Check sheet for the modelled part. Datum: model origin and axes. Units: mm. A direction names the side the tool comes from. Round coordinates to 2 decimals unless told otherwise and drop trailing zeros. Order: outer loops, then holes, each group sorted by start corner. A loop starts at its lowest first (then second) coordinate and runs counter-clockwise, first axis right, second up.
Q1. Cross-section at B-B on y = -62. Record the cut outline in (x, z).
Q2. Cross-section at D-D on y = -26. Record the cut outline in (x, z), then the cut area to 3 significant figures.
Q3. Set-up check for faces 4 (the flat face through (29, -14, 10)), 5 (the flat face through (98, 6, 2)), 6 (the cylindrical face through (-3.94, -45, -15.57)): record each of +Z, -Z, +X, -X, +Y, -Y from which the full face is reachable in a straight line by a thin tool's end or side.
Q4. Cross-section at A-A on x = 80.25. Record the cut outline in (y, z).
Q5. Scan lines: probe 1 along X at (y, z) = (8, 0); probe 2 along Z at (x, y) = (100.5, 4); probe 3 along X at (y, z) = (3, 9). Record each from-to range of solid material in increasing order.
Q6. Mould release check, pull along X, two halves, no side actions. Record for faces 1 (the flat face through (-4, -83, 0)), 2 (the cylindrical face through (-6.425, -33.544, -13.451)), 3 (the cylindrical face through (86.095, 7.521, -10.617)): +X half, -X half, draft (parallel to the pull), parting line (faces both ways), or undercut.
Q7. Depth check by flat-ended pin: P1, Ø15, axis at x = 37.5, y = -7.5, coming from the -Z side; P2, Ø3.5, axis at x = 90, z = -9.75, coming from the -Y side; P3, Ø12.5, axis at y = -70.5, z = -9.5, coming from the +X side. Enter the tip coordinate at first touch or a pass-through.
Q8. Cross-section at C-C on z = -15.5. Record the cut outline in (x, y), then the cut area to 3 significant figures.
from build123d import *

# Parameters (mm, degrees)
SKETCH_1_R           = 1.6
SKETCH_1_R_2         = 2.1
EXTRUDE_2_DEPTH      = 9
SKETCH_3_R           = 4
CUT_EXTRUDE_2_DEPTH  = 3
SKETCH_4_W           = 22.834782432
SKETCH_4_H           = 34.021608207
CUT_EXTRUDE_3_DEPTH  = 10
SKETCH_5_W           = 8
SKETCH_5_H           = 34
SKETCH_5_R           = 1.6
EXTRUDE_3_DEPTH      = 6
SKETCH_6_R           = 3.5
CUT_EXTRUDE_4_DEPTH  = 3
CUT_EXTRUDE_5_DEPTH  = 13
EXTRUDE_4_DEPTH      = 35
CUT_EXTRUDE_6_DEPTH  = 40
SKETCH_10_W          = 118.393769374
SKETCH_10_H          = 1
CUT_EXTRUDE_7_DEPTH  = 40
SKETCH_11_W          = 80.430163382
SKETCH_11_H          = 7.146133908
CUT_EXTRUDE_8_DEPTH  = 40
EXTRUDE_5_DEPTH      = 34
SKETCH_14_W          = 42
SKETCH_14_H          = 42
EXTRUDE_6_DEPTH      = 8
SKETCH_13_R          = 1.5
SKETCH_13_R_2        = 12
CUT_EXTRUDE_10_DEPTH = 8
SKETCH_15_W          = 89.303663432
SKETCH_15_H          = 7
SKETCH_15_H_2        = 10
EXTRUDE_7_DEPTH      = 4
FILLET_1_R           = 10
FILLET_2_R           = 10
FILLET_3_R           = 3


with BuildPart() as part:
    # 草图1 → 凸台-拉伸2 (new body)
    with BuildSketch(Plane(origin=(0, 0, 0), x_dir=(1, 0, 0), z_dir=(0, 1, 0))):
        with BuildLine():
            Line((0, 17), (90, 17))
            ThreePointArc((90, 17), (107, 0), (90, -17))
            Line((90, -17), (0, -17))
            ThreePointArc((0, -17), (-17, 0), (0, 17))
        make_face()
        with Locations(Location((90, 0, 0), (0, 0, 270))):
            Circle(SKETCH_1_R, mode=Mode.SUBTRACT)
        with Locations(Location((90, 9.75, 0), (0, 0, 270))):
            Circle(SKETCH_1_R, mode=Mode.SUBTRACT)
        with Locations(Location((99.75, 0, 0), (0, 0, 270))):
            Circle(SKETCH_1_R_2, mode=Mode.SUBTRACT)
        with Locations(Location((90, -9.75, 0), (0, 0, 270))):
            Circle(SKETCH_1_R, mode=Mode.SUBTRACT)
        with Locations(Location((80.25, 0, 0), (0, 0, 270))):
            Circle(SKETCH_1_R_2, mode=Mode.SUBTRACT)
    extrude(amount=EXTRUDE_2_DEPTH)

    # 草图3 → 切除-拉伸2 (cut)
    with BuildSketch(Plane(origin=(0, 9, 0), x_dir=(1, 0, 0), z_dir=(0, 1, 0))):
        with Locations(Location((90, 9.75, 0), (0, 0, 270))):
            Circle(SKETCH_3_R)
        with Locations(Location((99.75, 0, 0), (0, 0, 270))):
            Circle(SKETCH_3_R)
        with Locations(Location((90, -9.75, 0), (0, 0, 270))):
            Circle(SKETCH_3_R)
        with Locations(Location((80.25, 0, 0), (0, 0, 270))):
            Circle(SKETCH_3_R)
    extrude(amount=-CUT_EXTRUDE_2_DEPTH, mode=Mode.SUBTRACT)

    # 草图4 → 切除-拉伸3 (cut)
    with BuildSketch(Plane(origin=(0, 9, 0), x_dir=(1, 0, 0), z_dir=(0, 1, 0))):
        with Locations((-11.417391216, 0.010804103)):
            Rectangle(SKETCH_4_W, SKETCH_4_H)
    extrude(amount=-CUT_EXTRUDE_3_DEPTH, mode=Mode.SUBTRACT)

    # 草图5 → 凸台-拉伸3 (add)
    with BuildSketch(Plane(origin=(0, 9, 0), x_dir=(1, 0, 0), z_dir=(0, 1, 0))):
        with Locations((-4, 0)):
            Rectangle(SKETCH_5_W, SKETCH_5_H)
        with Locations(Location((-4, 10, 0), (0, 0, 270))):
            Circle(SKETCH_5_R, mode=Mode.SUBTRACT)
        with Locations(Location((-4, 0, 0), (0, 0, 270))):
            Circle(SKETCH_5_R, mode=Mode.SUBTRACT)
        with Locations(Location((-4, -10, 0), (0, 0, 270))):
            Circle(SKETCH_5_R, mode=Mode.SUBTRACT)
    extrude(amount=-EXTRUDE_3_DEPTH)

    # 草图6 → 切除-拉伸4 (cut)
    with BuildSketch(Plane(origin=(0, 9, 0), x_dir=(1, 0, 0), z_dir=(0, 1, 0))):
        with Locations(Location((-4, 10, 0), (0, 0, 270))):
            Circle(SKETCH_6_R)
        with Locations(Location((-4, 0, 0), (0, 0, 270))):
            Circle(SKETCH_6_R)
        with Locations(Location((-4, -10, 0), (0, 0, 270))):
            Circle(SKETCH_6_R)
    extrude(amount=-CUT_EXTRUDE_4_DEPTH, mode=Mode.SUBTRACT)

    # 草图7 → 切除-拉伸5 (cut)
    with BuildSketch(Plane(origin=(0, 9, 0), x_dir=(1, 0, 0), z_dir=(0, 1, 0))):
        with BuildLine():
            Line((68.25, -4), (7, -4))
            ThreePointArc((7, -4), (3, 0), (7, 4))
            Line((7, 4), (68.25, 4))
            ThreePointArc((68.25, 4), (72.25, 0), (68.25, -4))
        make_face()
    extrude(amount=-CUT_EXTRUDE_5_DEPTH, mode=Mode.SUBTRACT)

    # 草图8 → 凸台-拉伸4 (add)
    with BuildSketch(Plane.XY.offset(17)):
        Polygon((0, -83), (0, -41), (72.080145507, 0), (58.442959142, 0), (-8, -37.793504795), (-8, -41), (-8, -83), align=None)
    extrude(amount=-EXTRUDE_4_DEPTH)

    # 草图9 → 切除-拉伸6 (cut)
    with BuildSketch(Plane.XY.offset(17)):
        Polygon((58.442959142, 0), (68.123155874, 9), (-8, 9), (-8, 0), align=None)
    extrude(amount=-CUT_EXTRUDE_6_DEPTH, mode=Mode.SUBTRACT)

    # 草图10 → 切除-拉伸7 (cut)
    with BuildSketch(Plane(origin=(27.096230432, -29.144093474, 0), x_dir=(0.7323691027025148, 0.6809078479550029, 0), z_dir=(-0.6809078479550029, 0.7323691027025148, 0))):
        with Locations((-3.177419515, 17.5)):
            Rectangle(SKETCH_10_W, SKETCH_10_H)
    extrude(amount=-CUT_EXTRUDE_7_DEPTH, mode=Mode.SUBTRACT)

    # 草图11 → 切除-拉伸8 (cut)
    with BuildSketch(Plane(origin=(17.620285002, -30.977383092, 0), x_dir=(0.8692214499653501, 0.49442296763007937, 0), z_dir=(0.49442296763007937, -0.8692214499653501, 0))):
        with Locations((12.899580295, -20.573066954)):
            Rectangle(SKETCH_11_W, SKETCH_11_H)
    extrude(amount=-CUT_EXTRUDE_8_DEPTH, mode=Mode.SUBTRACT)

    # 草图12 → 凸台-拉伸5 (add)
    with BuildSketch(Plane.XY.offset(17)):
        Polygon((72.080145507, 0), (72.080145507, 9), (68.123155874, 9), (54.780591243, -2.083196181), (58.114256966, -7.94395497), align=None)
    extrude(amount=-EXTRUDE_5_DEPTH)

    # 草图14 → 凸台-拉伸6 (add)
    with BuildSketch(Plane.ZY.offset(8)):
        with Locations((0, -62)):
            Rectangle(SKETCH_14_W, SKETCH_14_H)
    extrude(amount=-EXTRUDE_6_DEPTH)

    # 草图13 → 切除-拉伸10 (cut)
    with BuildSketch(Plane(origin=(0, 0, 0), x_dir=(0, 0, -1), z_dir=(1, 0, 0))):
        with Locations(Location((-15.5, -46.5, 0), (0, 0, 90))):
            Circle(SKETCH_13_R)
        with Locations(Location((15.5, -46.5, 0), (0, 0, 270))):
            Circle(SKETCH_13_R)
        with Locations(Location((15.5, -77.5, 0), (0, 0, 90))):
            Circle(SKETCH_13_R)
        with Locations(Location((-15.5, -77.5, 0), (0, 0, 270))):
            Circle(SKETCH_13_R)
        with Locations(Location((0, -62, 0), (0, 0, 90))):
            Circle(SKETCH_13_R_2)
    extrude(amount=-CUT_EXTRUDE_10_DEPTH, mode=Mode.SUBTRACT)

    # 草图15 → 凸台-拉伸7 (add)
    with BuildSketch(Plane(origin=(14.286619279, -25.116624303, 0), x_dir=(0.86922144996535, 0.4944229676300795, 0), z_dir=(-0.4944229676300795, 0.86922144996535, 0))):
        with Locations((19.012083318, 13.5)):
            Rectangle(SKETCH_15_W, SKETCH_15_H)
        with Locations((19.012083318, 0)):
            Rectangle(SKETCH_15_W, SKETCH_15_H_2)
        with Locations((19.012083318, -13.5)):
            Rectangle(SKETCH_15_W, SKETCH_15_H)
    extrude(amount=EXTRUDE_7_DEPTH)

    # 圆角1
    # the kernel refuses this fillet: 10 mm, written as the material it takes off along each edge
    with BuildSketch(Plane(origin=(67.646967944, 9.837163299, -27.704780935), x_dir=(-0.8692214499653496, -0.4944229676300802, 0), z_dir=(0, 0, 1))) as fillet_1_piece_1:
        with BuildLine():
            CenterArc((4.281912374, 10), FILLET_1_R, 244.647173819, 25.352826181)
            Line((0, 0.963118546), (-0.085638247, 0.782380917))
            ThreePointArc((-0.085638247, 0.782380917), (-0.2, 0.481559273), (-0.2, 0))
            Line((-0.2, 0), (0, -0.2))
            Line((0, -0.2), (4.281912374, -0.2))
            Line((4.281912374, -0.2), (4.281912374, 0))
        make_face()
    extrude(amount=28.40956187, mode=Mode.SUBTRACT)
    with BuildSketch(Plane(origin=(67.646967944, 9.837163299, -15.704780935), x_dir=(-0.8692214499653494, -0.4944229676300803, 0), z_dir=(0, 0, 1))) as fillet_1_piece_2:
        with BuildLine():
            CenterArc((4.281912374, 10), FILLET_1_R, 244.647173819, 25.352826181)
            Line((0, 0.963118546), (-0.085638247, 0.782380917))
            ThreePointArc((-0.085638247, 0.782380917), (-0.2, 0.481559273), (-0.2, 0))
            Line((-0.2, 0), (0, -0.2))
            Line((0, -0.2), (4.281912374, -0.2))
            Line((4.281912374, -0.2), (4.281912374, 0))
        make_face()
    extrude(amount=31.40956187, mode=Mode.SUBTRACT)
    with BuildSketch(Plane(origin=(67.646967944, 9.837163299, 27.704780935), x_dir=(-0.8692214499653496, -0.4944229676300802, 0), z_dir=(0, 0, -1))) as fillet_1_piece_3:
        with BuildLine():
            CenterArc((4.281912374, -10), FILLET_1_R, 90, 25.352826181)
            Line((0, -0.963118546), (-0.085638247, -0.782380917))
            ThreePointArc((-0.085638247, -0.782380917), (-0.2, -0.481559273), (-0.2, 0))
            Line((-0.2, 0), (0, 0.2))
            Line((0, 0.2), (4.281912374, 0.2))
            Line((4.281912374, 0.2), (4.281912374, 0))
        make_face()
    extrude(amount=28.40956187, mode=Mode.SUBTRACT)
    with BuildSketch(Plane(origin=(-9.977691871, -34.316618995, 10), x_dir=(0.49442296763008015, -0.8692214499653496, 0), z_dir=(0, 0, -1))) as fillet_1_piece_4:
        with BuildLine():
            CenterArc((10, -8), FILLET_1_R, 126.869897646, 53.130102354)
            Line((0, -8), (-0.2, -8))
            Line((-0.2, -8), (-0.2, 0))
            Line((-0.2, 0), (0, 0.2))
            ThreePointArc((0, 0.2), (2, 0.2), (3.88, 0.16))
            Line((3.88, 0.16), (4, 0))
        make_face()
    extrude(amount=47, mode=Mode.SUBTRACT)
    with BuildSketch(Plane(origin=(-9.977691871, -34.316618995, 25), x_dir=(0.4944229676300804, -0.8692214499653496, 0), z_dir=(0, 0, -1))) as fillet_1_piece_5:
        with BuildLine():
            CenterArc((10, -8), FILLET_1_R, 126.869897646, 53.130102354)
            Line((0, -8), (-0.2, -8))
            Line((-0.2, -8), (-0.2, 0))
            Line((-0.2, 0), (0, 0.2))
            ThreePointArc((0, 0.2), (2, 0.2), (3.88, 0.16))
            Line((3.88, 0.16), (4, 0))
        make_face()
    extrude(amount=50, mode=Mode.SUBTRACT)
    with BuildSketch(Plane(origin=(-9.977691871, -34.316618995, -10), x_dir=(0.49442296763008015, -0.8692214499653496, 0), z_dir=(0, 0, 1))) as fillet_1_piece_6:
        with BuildLine():
            CenterArc((10, 8), FILLET_1_R, 180, 53.130102354)
            Line((0, 8), (-0.2, 8))
            Line((-0.2, 8), (-0.2, 0))
            Line((-0.2, 0), (0, -0.2))
            ThreePointArc((0, -0.2), (2, -0.2), (3.88, -0.16))
            Line((3.88, -0.16), (4, 0))
        make_face()
    extrude(amount=47, mode=Mode.SUBTRACT)

    # 圆角2
    # the kernel refuses this fillet: 10 mm, written as the material it adds along each edge
    with BuildSketch(Plane(origin=(72.080145507, 0, 17), x_dir=(-0.86922144996535, -0.4944229676300795, 0), z_dir=(0, 0, -1))) as fillet_2_piece_1_section:
        with BuildLine():
            CenterArc((FILLET_2_R * 0.264507433102, -FILLET_2_R), FILLET_2_R, 90, 29.631707367)
            Line((-FILLET_2_R * 0.229915534528, -FILLET_2_R * 0.130778550035), (0, 0))
            Line((0, 0), (FILLET_2_R * 0.264507433102, 0))
        make_face()
    fillet_2_piece_1 = extrude(amount=22.459435899, mode=Mode.PRIVATE)
    fillet_2_piece_1 = split(fillet_2_piece_1, bisect_by=Plane(origin=(72.080145507, -0.43196412, 9.594144242), z_dir=(-1, 0, 0)), keep=Keep.TOP, mode=Mode.PRIVATE)
    add(fillet_2_piece_1)
    with BuildSketch(Plane(origin=(72.080145507, 0, 17), x_dir=(-0.86922144996535, -0.4944229676300795, 0), z_dir=(0, 0, -1))) as fillet_2_piece_2_section:
        with BuildLine():
            CenterArc((FILLET_2_R * 0.264507433102, -FILLET_2_R), FILLET_2_R, 90, 29.631707367)
            Line((-FILLET_2_R * 0.229915534528, -FILLET_2_R * 0.130778550035), (0, 0))
            Line((0, 0), (FILLET_2_R * 0.264507433102, 0))
        make_face()
    fillet_2_piece_2 = extrude(amount=22.459435899, mode=Mode.PRIVATE)
    fillet_2_piece_2 = fillet_2_piece_2 - Plane(origin=(68.25, -0.105711956, 0), x_dir=(0, 0, -1), z_dir=(0, 1, 0)) * Cylinder(4, 56, mode=Mode.PRIVATE)
    add(fillet_2_piece_2)
    with BuildSketch(Plane(origin=(72.080145507, 0, 5.459435899), x_dir=(-0.86922144996535, -0.4944229676300795, 0), z_dir=(0, 0, -1))) as fillet_2_piece_3_section:
        with BuildLine():
            CenterArc((FILLET_2_R * 0.264507433102, -FILLET_2_R), FILLET_2_R, 90, 29.631707367)
            Line((-FILLET_2_R * 0.229915534528, -FILLET_2_R * 0.130778550035), (0, 0))
            Line((0, 0), (FILLET_2_R * 0.264507433102, 0))
        make_face()
    fillet_2_piece_3 = extrude(amount=22.459435899, mode=Mode.PRIVATE)
    fillet_2_piece_3 = split(fillet_2_piece_3, bisect_by=Plane(origin=(72.080145507, -0.402309052, 3.779769442), z_dir=(-1, 0, 0)), keep=Keep.TOP, mode=Mode.PRIVATE)
    add(fillet_2_piece_3)
    with BuildSketch(Plane(origin=(72.080145507, 0, 5.459435899), x_dir=(-0.86922144996535, -0.4944229676300795, 0), z_dir=(0, 0, -1))) as fillet_2_piece_4_section:
        with BuildLine():
            CenterArc((FILLET_2_R * 0.264507433102, -FILLET_2_R), FILLET_2_R, 90, 29.631707367)
            Line((-FILLET_2_R * 0.229915534528, -FILLET_2_R * 0.130778550035), (0, 0))
            Line((0, 0), (FILLET_2_R * 0.264507433102, 0))
        make_face()
    fillet_2_piece_4 = extrude(amount=22.459435899, mode=Mode.PRIVATE)
    fillet_2_piece_4 = fillet_2_piece_4 - Plane(origin=(68.25, -0.105711956, 0), x_dir=(0, 0, -1), z_dir=(0, 1, 0)) * Cylinder(4, 56, mode=Mode.PRIVATE)
    add(fillet_2_piece_4)

    # 圆角3
    fillet_3_edges = [part.edges().sort_by_distance(p)[0] for p in [
        (-4, -83, 21),
        (-4, -41, 21),
        (-4, -83, -21),
        (-4, -41, -21),
    ]]
    fillet(fillet_3_edges, radius=FILLET_3_R)


solid = part.part
Results found:
1. outline: (-8, -21) - (0, -21) - (0, -12) - (-8, -12) - close; (-8, 12) - (0, 12) - (0, 21) - (-8, 21) - close
2. outline: (4.64, -17) - (26.37, -17) - (26.37, 17) - (4.64, 17) - (4.64, 10) - (12.73, 10) - (12.73, 5) - (4.64, 5) - (4.64, -5) - (12.73, -5) - (12.73, -10) - (4.64, -10) - close
2. area: 658 mm2
3. face 4: -X, +Y
3. face 5: +Y
3. face 6: +X, -X
4. outline: (0, -17) - (9, -17) - (9, -4) - (6, -4) - (6, -2.1) - (0, -2.1) - close; (0, 2.1) - (6, 2.1) - (6, 4) - (9, 4) - (9, 17) - (0, 17) - close
5. probe 1: x = 64.45 to 72.08, 72.25 to 76.25, 84.25 to 88.4, 91.6 to 95.75, 103.75 to 107
5. probe 2: z = -13.37 to -1.96, 1.96 to 13.37
5. probe 3: x = 60.9 to 88.59, 91.41 to 104.42
6. face 1: draft
6. face 2: -X half
6. face 3: undercut
7. P1: stops at z = -17
7. P2: stops at y = 0
7. P3: stops at x = 0
8. outline: (-8, -83) - (0, -83) - (0, -79) - (-8, -79) - close; (-8, -76) - (0, -76) - (0, -48) - (-8, -48) - close; (-8, -45) - (0, -45) - (0, -41) - (69.78, -1.31) arc R10 cw to (74.73, 0) - (96.98, 0) - (96.98, 9) - (68.12, 9) arc R10 ccw to (63.93, 7.72) - (-3.02, -30.36) arc R10 ccw to (-8, -37.79) - close
8. area: 1,470 mm2
